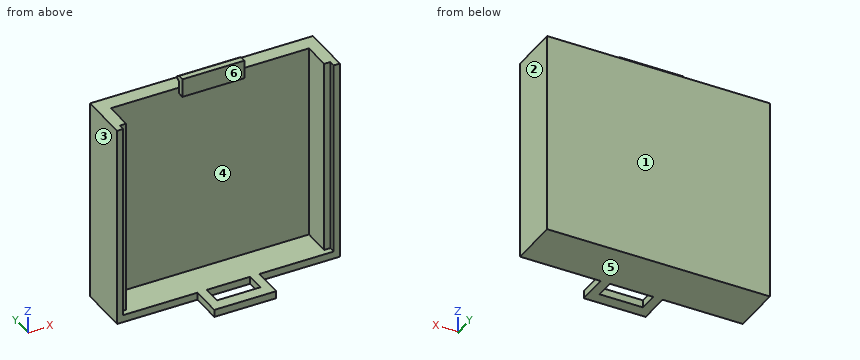
from build123d import *

# Parameters (mm, degrees)
SALIENTE_EXTRUIR1_DEPTH      = 33
SALIENTE_EXTRUIR2_DEPTH      = 1.2
SALIENTE_EXTRUIR3_DEPTH      = 1.2
SALIENTE_EXTRUIR4_DEPTH      = 2
SALIENTE_EXTRUIR4_DEPTH_BACK = 1
CROQUIS4_W                   = 10
CROQUIS4_H                   = 1
SALIENTE_EXTRUIR5_DEPTH      = 10


with BuildPart() as part:
    # Croquis1 → Saliente-Extruir1 (new body)
    with BuildSketch(Plane.XY):
        Polygon((-18, -5.5), (-17, -5.5), (-17, -4.5), (-16, -4.5), (-16, 0), (16, 0), (16, -4.5), (17, -4.5), (17, -5.5), (18, -5.5), (18, 2.5), (-18, 2.5), align=None)
    extrude(amount=SALIENTE_EXTRUIR1_DEPTH)

    # Croquis2 → Saliente-Extruir2 (add)
    with BuildSketch(Plane.XY):
        Polygon((17, -5.5), (-17, -5.5), (-17, -4.5), (-16, -4.5), (-16, 0), (16, 0), (16, -4.5), (17, -4.5), align=None)
    extrude(amount=SALIENTE_EXTRUIR2_DEPTH)

    # Croquis3 → Saliente-Extruir3 (add)
    with BuildSketch(Plane.XY):
        Polygon((5, -5.5), (5, -10.5), (-5, -10.5), (-5, -5.5), (-3.5, -5.5), (-3.5, -8.55), (3.5, -8.55), (3.5, -5.5), align=None)
    extrude(amount=SALIENTE_EXTRUIR3_DEPTH)

    # Croquis4 → Saliente-Extruir4 (add, two sides: drawn at the far end of the back side and taken through both)
    with BuildSketch(Plane.XY.offset(33).offset(-SALIENTE_EXTRUIR4_DEPTH_BACK)):
        with Locations((0, -0.5)):
            Rectangle(CROQUIS4_W, CROQUIS4_H)
    extrude(amount=SALIENTE_EXTRUIR4_DEPTH + SALIENTE_EXTRUIR4_DEPTH_BACK)

    # Croquis5 → Saliente-Extruir5 (add)
    with BuildSketch(Plane(origin=(5, 0, 0), x_dir=(0, 0, -1), z_dir=(1, 0, 0))):
        Polygon((-35, 0), (-34.5, 0.7), (-34, 0), align=None)
    extrude(amount=-SALIENTE_EXTRUIR5_DEPTH)


solid = part.part
The listing builds one solid part. Answer for the finished solid, in the listing's coordinates (mm). Face numbers are marked on the shaded views. A direction names the side the tool comes from. Coordinates: 2 decimals unless noted, no trailing zeros. Order: outer loops, then holes, each group sorted by start corner. A loop starts at its lowest first (then second) coordinate and runs counter-clockwise, first axis right, second up. Notation, with made-up numbers: (19, -32) -> (57, -32) arc R7 cw to (57, -25) -> close; hole circle Ø4 at (59.25, 55.5). An arc over 180 degrees is marked (long way). Answer in a Markdown table with one row per item. Add a question column.
Item 1: Which of the six approach directions +Z, -Z, +X, -X, +Y, -Y give full straight-line access (tool end or side, diameter ignored) to the marked faces 5 and 6?
Item 2: Find the intervals of material crossed by L1, parallel to X at y = -5, z = 31; L2, parallel to X at y = -3.75, z = 11; L3, parallel to Y at x = -12, z = 4, in increasing order. Write a range as from..to.
Item 3: Find section C-C (x = 4). Write down the section's boundary in (y, z).
Item 4: Determine the mould class of the marked faces 1, 2, 3 and 4 for opening direction X: +X half, -X half, draft (parallel to the pull), parting line (faces both ways), or undercut.
Item 5: Find section A-A (x = -2). Write down the section's boundary in (y, z).
Item 6: Find section D-D (z = 21.5). Write down the section's boundary in (x, y).
Item 7: Each of these flat-tipped pins is pushed along its axis until it touches: P1, Ø0.5, axis at x = -2, z = 33.5, coming from the +Y side; P2, Ø1.4, axis at y = 0, z = 34, coming from the +X side; P3, Ø2.5, axis at x = 7, y = -2, coming from the +Z side. Where does it stop, or does it pass through?
Item 8: Find section B-B (y = -7). Write down the section's boundary in (x, z).
Result set:
| question | item | result |
|---|---|---|
| 1 | face 5 | -Z, +X, -X, +Y, -Y |
| 1 | face 6 | +Z, -Y |
| 2 | L1 | x = -18..-17, 17..18 |
| 2 | L2 | x = -18..-16, 16..18 |
| 2 | L3 | y = 0..2.5 |
| 3 | outline | (-10.5, 0) -> (2.5, 0) -> (2.5, 33) -> (0, 33) -> (0, 34) -> (0.7, 34.5) -> (0, 35) -> (-1, 35) -> (-1, 32) -> (0, 32) -> (0, 1.2) -> (-10.5, 1.2) -> close |
| 4 | face 1 | draft |
| 4 | face 2 | +X half |
| 4 | face 3 | -X half |
| 4 | face 4 | undercut |
| 5 | outline | (-10.5, 0) -> (-8.55, 0) -> (-8.55, 1.2) -> (-10.5, 1.2) -> close; (-5.5, 0) -> (2.5, 0) -> (2.5, 33) -> (0, 33) -> (0, 34) -> (0.7, 34.5) -> (0, 35) -> (-1, 35) -> (-1, 32) -> (0, 32) -> (0, 1.2) -> (-5.5, 1.2) -> close |
| 6 | outline | (-18, -5.5) -> (-17, -5.5) -> (-17, -4.5) -> (-16, -4.5) -> (-16, 0) -> (16, 0) -> (16, -4.5) -> (17, -4.5) -> (17, -5.5) -> (18, -5.5) -> (18, 2.5) -> (-18, 2.5) -> close |
| 7 | P1 | stops at y = 0 |
| 7 | P2 | stops at x = 5 |
| 7 | P3 | stops at z = 1.2 |
| 8 | outline | (-5, 0) -> (-3.5, 0) -> (-3.5, 1.2) -> (-5, 1.2) -> close; (3.5, 0) -> (5, 0) -> (5, 1.2) -> (3.5, 1.2) -> close |
